```python
from build123d import *

# Parameters (mm, degrees)
F0_R     = 4.0005
F0_R_2   = 2.4765
F0_R_3   = 12.7
F0_R_4   = 5.08
F1_DEPTH = 3.03784


with BuildPart() as f1:
    # F0 (on Top) → F1 (new body)
    with BuildSketch(Plane.XY):
        Polygon((-97.120928, -190.5), (290.385188, 0), (-97.120928, 190.5), align=None)
        with Locations((-8.474928, -32.004)):
            Circle(F0_R, mode=Mode.SUBTRACT)
        with Locations((55.533072, -32.004)):
            Circle(F0_R, mode=Mode.SUBTRACT)
        with Locations((88.832472, -23.5458)):
            Circle(F0_R_2, mode=Mode.SUBTRACT)
        with Locations((135.974872, -23.5458)):
            Circle(F0_R_2, mode=Mode.SUBTRACT)
        with Locations((-8.474928, 32.004)):
            Circle(F0_R, mode=Mode.SUBTRACT)
        with Locations((23.529072, 0)):
            Circle(F0_R_3, mode=Mode.SUBTRACT)
        with Locations((88.832472, 23.5966)):
            Circle(F0_R_2, mode=Mode.SUBTRACT)
        with Locations((55.533072, 32.004)):
            Circle(F0_R, mode=Mode.SUBTRACT)
        with Locations((112.429072, 0)):
            Circle(F0_R_4, mode=Mode.SUBTRACT)
        with Locations((135.974872, 23.5966)):
            Circle(F0_R_2, mode=Mode.SUBTRACT)
    extrude(amount=F1_DEPTH)


solid = f1.part
```
Source: CAD feature listing. Evaluate the final solid. Frame: model axes, mm. Coordinates: 2 decimals unless noted, no trailing zeros. Loops run counter-clockwise (first coordinate to the right, second up) from the corner with the lowest first, then second, coordinate; pieces in that order, holes last. Notation, with made-up numbers: M 64.25,31.25 L 90.25,31.25 A24 cw 90.25,63.25 Z; hole C -36.75,4 d3. An arc over 180 degrees is marked long. Use a Markdown table: item, result. Add a question column.
Q1. Material intervals for L1, parallel to X at y = -25, z = 1.4; L2, parallel to Y at x = -12, z = 1.8; L3, parallel to X at y = -11.5, z = 2.35, sorted ascending.
Q2. Section query B-B, the plane x = 147.5. Return loops of the section in (y, z), and give its area (3 significant figures).
Q3. First-contact query: pin 1 (1.5 mm diameter, centred on y = 114.5, z = 1, fed in from +X). Flat tip, straight axial feed; report the tip coordinate or a pass-through.
Q4. Section query A-A, the plane z = 2. State how many separate pieces and enclosed holes the cut face has, and give its area (3 significant figures).
Q5. Draft query along X for faces 1 (the flat face through (51, 3, 3.038)), 2 (the cylindrical face through (117.274, 1.526, 1.498)), 3 (the flat face through (99.34, 93.92, 1.5)). Return one class per face: pulls with the +X half, pulls with the -X half, needs draft (parallel to the pull), parting line crosses it, or undercut.
Q6. Section query C-C, the plane y = -76. Return loops of the section in (x, z).
Result:
| question | item | result |
|---|---|---|
| 1 | L1 | x = -97.12 to 86.83, 90.84 to 133.97, 137.98 to 239.53 |
| 1 | L2 | y = -148.65 to -33.9, -30.11 to 30.11, 33.9 to 148.65 |
| 1 | L3 | x = -97.12 to 18.14, 28.92 to 266.99 |
| 2 | outline | M -70.24,0 L 70.24,0 L 70.24,3.04 L -70.24,3.04 Z |
| 2 | area | 427 mm2 |
| 3 | pin 1 | stops at x = 59 |
| 4 | separate pieces | 1 |
| 4 | enclosed holes | 10 |
| 4 | area | 73,000 mm2 |
| 5 | face 1 | needs draft |
| 5 | face 2 | undercut |
| 5 | face 3 | pulls with the +X half |
| 6 | outline | M -97.12,0 L 135.79,0 L 135.79,3.04 L -97.12,3.04 Z |
